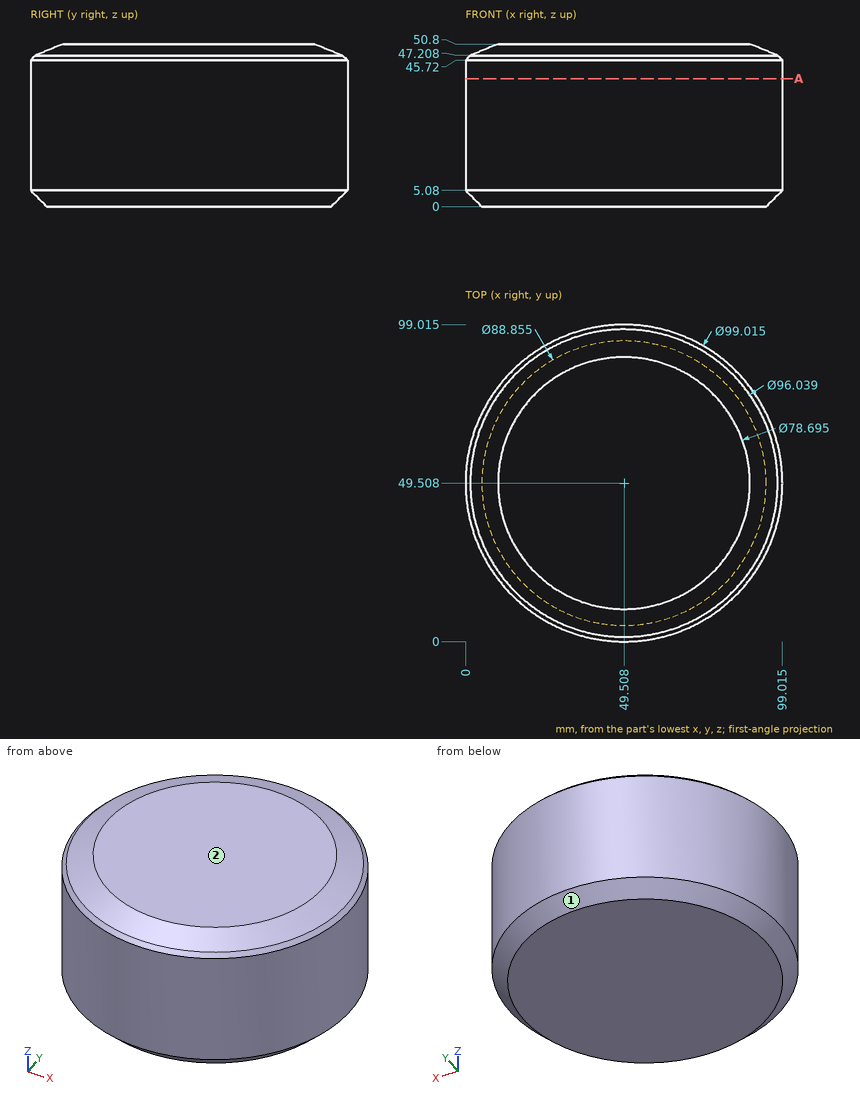
Answer from the drawing. Dimensions are ordinates in mm from the lowest x, y and z of the part. Give positions to 0.01 mm unless a question says otherwise; leave off trailing zeros. Loops run counter-clockwise (first coordinate to the right, second up) from the corner with the lowest first, then second, coordinate; pieces in that order, holes last. Notation, with made-up numbers: (-33, 31.5) -> (-2, 31.5) arc R4 ccw to (-2, 35.5) -> close; hole circle Ø5 at (-14.75, -0.75). An arc over 180 degrees is marked (long way). One line per question, with ' | ' between items. Start each with the question number.
1) Straight lines are drawn through the part: L1, parallel to Z at x = 77.5, y = 13 (1 decimal); L2, parallel to Y at x = 10.5, z = 37 (1 decimal); L3, parallel to Z at x = 69.5, y = 94.5 (1 decimal). For each, find the intervals that lie inside material, in ascending order.
2) Determine the mould class of the marked faces 1 and 2 for opening direction X: +X half, -X half, draft (parallel to the pull), parting line (faces both ways), or undercut.
3) Section A-A, the plane z = 40 is taken. Determine the outline of the cut face in (x, y) (1 decimal).
4) Each of these flat-tipped pins is pushed along its axis until it touches: pin 1 (8 mm diameter, centred on x = 20, z = 6.5, fed in from +Y); pin 2 (1.5 mm diameter, centred on x = 48.5, z = 15, fed in from +Y); pin 3 (10 mm diameter, centred on y = 37, z = 43, fed in from -X). Where does it stop, or does it pass through?
Resolved:
1) L1: 1.6 to 48 | L2: 19 to 80 | L3: 4.8 to 46
2) face 1: parting line | face 2: draft
3) outline: circle Ø99 at (49.5, 49.5)
4) pin 1: y = 91.94 | pin 2: y = 99.01 | pin 3: x = 0.57
